```python
from build123d import *

# Parameters (mm, degrees)
F0_R     = 5.6
F0_W     = 30
F0_H     = 15
F1_DEPTH = 5


with BuildPart() as f1:
    # F0 (on Front) → F1 (new body, symmetric)
    with BuildSketch(Plane.XZ):
        Polygon((50, 7.5), (-50, 7.5), (-50, -7.5), (-20, -7.5), (20, -7.5), (50, -7.5), align=None)
        with Locations((-34, 0)):
            Circle(F0_R, mode=Mode.SUBTRACT)
        with Locations((34, 0)):
            Circle(F0_R, mode=Mode.SUBTRACT)
        with Locations((-35, -15)):
            Rectangle(F0_W, F0_H)
        with Locations((35, -15)):
            Rectangle(F0_W, F0_H)
    extrude(amount=F1_DEPTH, both=True)


solid = f1.part
```
Build history of the part. All positions in model axes, mm. A direction names the side the tool comes from. Round coordinates to 2 decimals unless told otherwise and drop trailing zeros. Write each loop counter-clockwise with the first axis right and the second up, starting at its lowest first coordinate (ties: lowest second). Pieces come first, ordered by that corner, then holes. Notation, with made-up numbers: (24.25, 13) -> (66.25, 13) arc R25 ccw to (66.25, 25) -> close; hole circle Ø4 at (44, 78). An arc over 180 degrees is marked (long way). Put each result on its own line as item: value.
Item 1: Two-plate mould, pull along X, no slides. Class faces 3 (the face through (-50, 0, -7)), 4 (the face through (-1, -5, -7)), 5 (the face through (20, 0, -15)): pulls with the +X half, pulls with the -X half, needs draft (parallel to the pull), parting line crosses it, or undercut.
Here are the results:
face 3: pulls with the -X half
face 4: needs draft
face 5: undercut
Item 2: Slice it at B-B, the plane x = 34. Give the cut face in (y, z), plus the area to 3 significant figures.
Here are the results:
outline: (-5, -22.5) -> (5, -22.5) -> (5, -5.6) -> (-5, -5.6) -> close; (-5, 5.6) -> (5, 5.6) -> (5, 7.5) -> (-5, 7.5) -> close
area: 188 mm^2
Item 3: Flat gauge pin, fed straight in: P1, Ø5, axis at x = 5.5, y = 0.5, coming from the -Z side. Where does the tip first touch, or does it go through?
Here are the results:
P1: stops at z = -7.5
Item 4: Slice it at A-A, the plane y = 1.5. Give the cut face in (x, z).
Here are the results:
outline: (-50, -22.5) -> (-20, -22.5) -> (-20, -7.5) -> (20, -7.5) -> (20, -22.5) -> (50, -22.5) -> (50, 7.5) -> (-50, 7.5) -> close; hole circle Ø11.2 at (-34, 0); hole circle Ø11.2 at (34, 0)
Item 5: Slice it at D-D, the plane z = 0. Give the cut face in (x, y).
Here are the results:
outline: (-50, -5) -> (-39.6, -5) -> (-39.6, 5) -> (-50, 5) -> close; (-28.4, -5) -> (28.4, -5) -> (28.4, 5) -> (-28.4, 5) -> close; (39.6, -5) -> (50, -5) -> (50, 5) -> (39.6, 5) -> close
Item 6: Tool access for faces 1 (the face through (35, 0, -22.5)), 2 (the face through (-20, 0, -15)): list every direction of +Z, -Z, +X, -X, +Y, -Y with a clear straight run to the whole face (end or side of a thin tool).
Here are the results:
face 1: -Z, +X, -X, +Y, -Y
face 2: -Z, +Y, -Y
Item 7: Slice it at C-C, the plane z = -20.5. Give the cut face in (x, y), plus the area to 3 significant figures.
Here are the results:
outline: (-50, -5) -> (-20, -5) -> (-20, 5) -> (-50, 5) -> close; (20, -5) -> (50, -5) -> (50, 5) -> (20, 5) -> close
area: 600 mm^2
Item 8: Wall check: probe 1 along X at (y, z) = (-1.5, -13); probe 2 along Z at (x, y) = (-34, 0); probe 3 along X at (y, z) = (3.5, -5). Give the ranges that are in metal, low to high. Write a range as from..to.
Here are the results:
probe 1: x = -50..-20, 20..50
probe 2: z = -22.5..-5.6, 5.6..7.5
probe 3: x = -50..-36.52, -31.48..31.48, 36.52..50
